```python
from build123d import *

# Parameters (mm, degrees)
SKETCH1_W           = 100
SKETCH1_H           = 100
BOSS_EXTRUDE1_DEPTH = 15
SKETCH2_R           = 4.65
CUT_EXTRUDE1_DEPTH  = 73.284161474
SKETCH10_R          = 5.9
CUT_EXTRUDE5_DEPTH  = 73.284161474
FILLET1_R           = 20
FILLET2_R           = 15


with BuildPart() as part:
    # Sketch1 → Boss-Extrude1 (new body)
    with BuildSketch(Plane.XY):
        Rectangle(SKETCH1_W, SKETCH1_H)
    extrude(amount=BOSS_EXTRUDE1_DEPTH)

    # Sketch2 → Cut-Extrude1 (cut, through all)
    with BuildSketch(Plane.XY.offset(15)):
        with Locations((35, 35)):
            Circle(SKETCH2_R)
        with Locations(Location((-35, -35, 0), (0, 0, 180))):
            Circle(SKETCH2_R)
    extrude(amount=-CUT_EXTRUDE1_DEPTH, mode=Mode.SUBTRACT)

    # Sketch10 → Cut-Extrude5 (cut, through all)
    with BuildSketch(Plane.XY.offset(15)):
        Circle(SKETCH10_R)
    extrude(amount=-CUT_EXTRUDE5_DEPTH, mode=Mode.SUBTRACT)

    # Fillet1
    fillet1_edges = [part.edges().sort_by_distance(p)[0] for p in [
        (-50, 50, 7.5),
        (50, -50, 7.5),
    ]]
    fillet(fillet1_edges, radius=FILLET1_R)

    # Fillet2
    fillet2_edges = [part.edges().sort_by_distance(p)[0] for p in [
        (50, 50, 7.5),
        (-50, -50, 7.5),
    ]]
    fillet(fillet2_edges, radius=FILLET2_R)


solid = part.part
```
Geometry check sheet. Reference: the model listing, model coordinates, mm. Round coordinates to 2 decimals unless told otherwise and drop trailing zeros. Order: outer loops, then holes, each group sorted by start corner. A loop starts at its lowest first (then second) coordinate and runs counter-clockwise, first axis right, second up. Notation, with made-up numbers: M 43.25,-8.5 L 100.25,-8.5 A18 cw 100.25,26.5 Z; hole C -22.5,28.25 d7. An arc over 180 degrees is marked long. Answer as CSV lines item,"result".
1) Sectioned sample at A-A on y = 0. Record the cut outline in (x, z).
Entries:
outline,"M -50,0 L -5.9,0 L -5.9,15 L -50,15 Z; M 5.9,0 L 50,0 L 50,15 L 5.9,15 Z"
2) Thickness scan on probe 1 along Y at (x, z) = (-0.5, 1.75); probe 2 along Y at (x, z) = (35, 3.5); probe 3 along X at (y, z) = (31, 14). Record the ranges inside material, lowest first. Write a range as [from, to].
Entries:
probe 1,"[-50, -5.88], [5.88, 50]"
probe 2,"[-49.36, 30.35], [39.65, 50]"
probe 3,"[-49.97, 32.63], [37.37, 50]"
3) Sectioned sample at C-C on z = 7. Record the cut outline in (x, y).
Entries:
outline,"M -50,-35 A15 ccw -35,-50 L 30,-50 A20 ccw 50,-30 L 50,35 A15 ccw 35,50 L -30,50 A20 ccw -50,30 Z; hole C -35,-35 d9.3; hole C 0,0 d11.8; hole C 35,35 d9.3"
4) Gauge pin test, flat end, axial feed: pin 1 Ø1.5 at (y, z) = (36, 7) entering from -X. Record the tip position at first contact, or that the pin passes through.
Entries:
pin 1,"x = -49.3"
5) Sectioned sample at D-D on x = 43. Record the cut outline in (y, z).
Entries:
outline,"M -45.2,0 L 47.69,0 L 47.69,15 L -45.2,15 Z"
6) Mould release check, pull along Y, two halves, no side actions. Record for faces 1 (the face through (37.5, 38.92, 7.6)), 2 (the face through (-3, -50, 7)), 3 (the face through (-37.5, -38.92, 7.6)), 4 (the face through (45.49, 45.72, 7.6)): +Y half, -Y half, draft (parallel to the pull), parting line (faces both ways), or undercut.
Entries:
face 1,"undercut"
face 2,"-Y half"
face 3,"undercut"
face 4,"+Y half"
